Verification items for the finished model (mm, model axes). Face numbers are marked on the shaded views. A direction names the side the tool comes from. Coordinates: 2 decimals unless noted, no trailing zeros. Write each loop counter-clockwise with the first axis right and the second up, starting at its lowest first coordinate (ties: lowest second). Pieces come first, ordered by that corner, then holes. Notation, with made-up numbers: M -18.5,11.5 L 27.5,11.5 A25 ccw 27.5,32.5 Z; hole C -9,87.5 d8. An arc over 180 degrees is marked long. One line per item, written item: value.
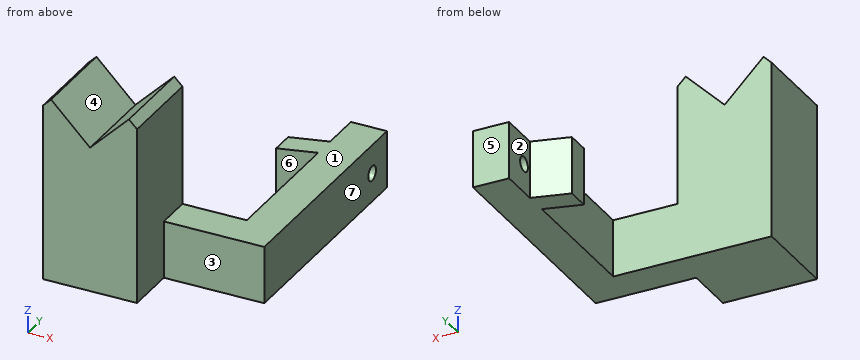
```python
from build123d import *

# Parameters (mm, degrees)
F0_W          = 44.45
F0_H          = 12.7
F1_DEPTH      = 8.001
F3_DEPTH      = 7.9375
F5_DEPTH      = 7.9375
F5_DEPTH_BACK = 11.43
F6_R          = 1.651
F7_DEPTH      = 25.4
F9_DEPTH      = 12.7


with BuildPart() as f1:
    # F0 (on Right) → F1 (new body)
    with BuildSketch(Plane.YZ):
        with Locations((-22.225, 6.35)):
            Rectangle(F0_W, F0_H)
    extrude(amount=F1_DEPTH)

    # F2 (on face) → F3 (join)
    with BuildSketch(Plane.XZ.offset(44.45)):
        Polygon((8.001, 12.7), (0, 12.7), (-35.08248, 12.7), (-35.08248, 0), (0, 0), (8.001, 0), align=None)
    extrude(amount=F3_DEPTH)

    # F4 (on face) → F5 (join, two sides)
    with BuildSketch(Plane.XZ.offset(52.3875)) as f5_sk:
        Polygon((-35.08248, 39.1567536341), (-35.08248, 0), (-14.25448, 0), (-14.25448, 39.1567536341), (-16.0505312242, 40.9528048583), (-24.66848, 32.3348560825), (-33.2864287758, 40.9528048583), align=None)
    extrude(amount=-F5_DEPTH)
    extrude(f5_sk.sketch, amount=F5_DEPTH_BACK)

    # F6 (on face) → F7 (cut)
    with BuildSketch(Plane.YZ.offset(8.001)):
        with Locations((-6.35, 6.35)):
            Circle(F6_R)
    extrude(amount=-F7_DEPTH, mode=Mode.SUBTRACT)

    # F8 (on face) → F9 (join, through all)
    with BuildSketch(Plane(origin=(0, 0, 0), x_dir=(1, 0, 0), z_dir=(0, 0, -1))):
        Polygon((-8.1650869207, 11.0778284465), (0, 8.89), (0, 13.97), (-8.1650869207, 16.1578284465), align=None)
    extrude(amount=-F9_DEPTH)


solid = f1.part
```
Item 1: Go/stop test with flat-tipped pins: P1, Ø5.5, axis at y = -12.5, z = 5, coming from the -X side; P2, Ø14, axis at y = -25, z = 9, coming from the -X side; P3, Ø10, axis at x = -3.5, y = -40, coming from the +Z side. Record where each tip stops, or that it passes through.
The answers:
P1: stops at x = -8.17
P2: stops at x = 0
P3: stops at z = 12.7
Item 2: Cross-section at A-A, the plane y = -6.35. Enter the section's corners in (x, z).
The answers:
outline: M 0,0 L 8,0 L 8,4.7 L 0,4.7 Z; M 0,8 L 8,8 L 8,12.7 L 0,12.7 Z
Item 3: Cross-section at C-C, the plane x = 3.5. Enter the section's corners in (y, z).
The answers:
outline: M -52.39,0 L 0,0 L 0,12.7 L -52.39,12.7 Z; hole C -6.35,6.35 d3.3
Item 4: Cross-section at D-D, the plane y = -39. Enter the section's corners in (x, z).
The answers:
outline: M 0,0 L 8,0 L 8,12.7 L 0,12.7 Z
Item 5: Draft check along X on the marked faces 4, 5, 6 and 7. Enter one of: released by +X, released by -X, zero draft, split by the parting line, or undercut.
The answers:
face 4: undercut
face 5: zero draft
face 6: undercut
face 7: released by +X
Item 6: Cross-section at B-B, the plane z = 6.35. Enter the section's corners in (x, y).
The answers:
outline: M -35.08,-63.82 L -14.25,-63.82 L -14.25,-52.39 L 8,-52.39 L 8,-8 L 0,-8 L 0,-8.89 L -8.17,-11.08 L -8.17,-16.16 L 0,-13.97 L 0,-44.45 L -35.08,-44.45 Z; M 0,-4.7 L 8,-4.7 L 8,0 L 0,0 Z
Item 7: Access from +Z, -Z, +X, -X, +Y, -Y to the whole of each face (thin tool, end or side, straight path). Record for the marked faces 1, 2 and 3.
The answers:
face 1: +Z, +X, +Y, -Y
face 2: +Z, -Z, -X, +Y
face 3: +Z, -Z, +X, -Y
Item 8: Scan lines: line 1 (Z direction, x = 4.75, y = -6.35); line 2 (Y direction, x = -24.5, z = 16.5); line 3 (Z direction, x = -4, y = -13). Record each from-to range of solid material in increasing order.
The answers:
line 1: z = 0 to 4.7, 8 to 12.7
line 2: y = -63.82 to -44.45
line 3: z = 0 to 12.7
